Check sheet for the drawn part. Datum: minimum x, y, z corner. Units: mm. Coordinates: 2 decimals unless noted, no trailing zeros. Loops run counter-clockwise (first coordinate to the right, second up) from the corner with the lowest first, then second, coordinate; pieces in that order, holes last.
Q1. Sectioned sample at C-C (y = 7.5). Count the separate pieces of the cut face and the enclosed holes in it, then the cut area to 3 significant figures.
Q2. Material ranges on probe 1 along Z at (x, y) = (135, 7) (1 decimal); probe 2 along X at (y, z) = (9.5, 160) (1 decimal); probe 3 along Z at (x, y) = (17.5, 6.5), recorded low to high.
Q3. Sectioned sample at B-B (z = 25). Enter the section's corners in (x, y) (1 decimal), then the cut area to 3 significant figures.
Q4. Sectioned sample at D-D (x = 217). Enter the section's corners in (y, z), then the cut area to 3 significant figures.
Q5. Sectioned sample at A-A (x = 135). Enter the section's corners in (y, z) (1 decimal), then the cut area to 3 significant figures.
Q6. Go/stop test with flat-tipped pins: P1, Ø6, axis at x = 189, y = 5.5, coming from the +Z side; P2, Ø1.5, axis at y = 2, z = 192.5, coming from the -X side; P3, Ø3, axis at x = 69, y = 5.5, coming from the +Z side. Record where each tip stops, or that it passes through.
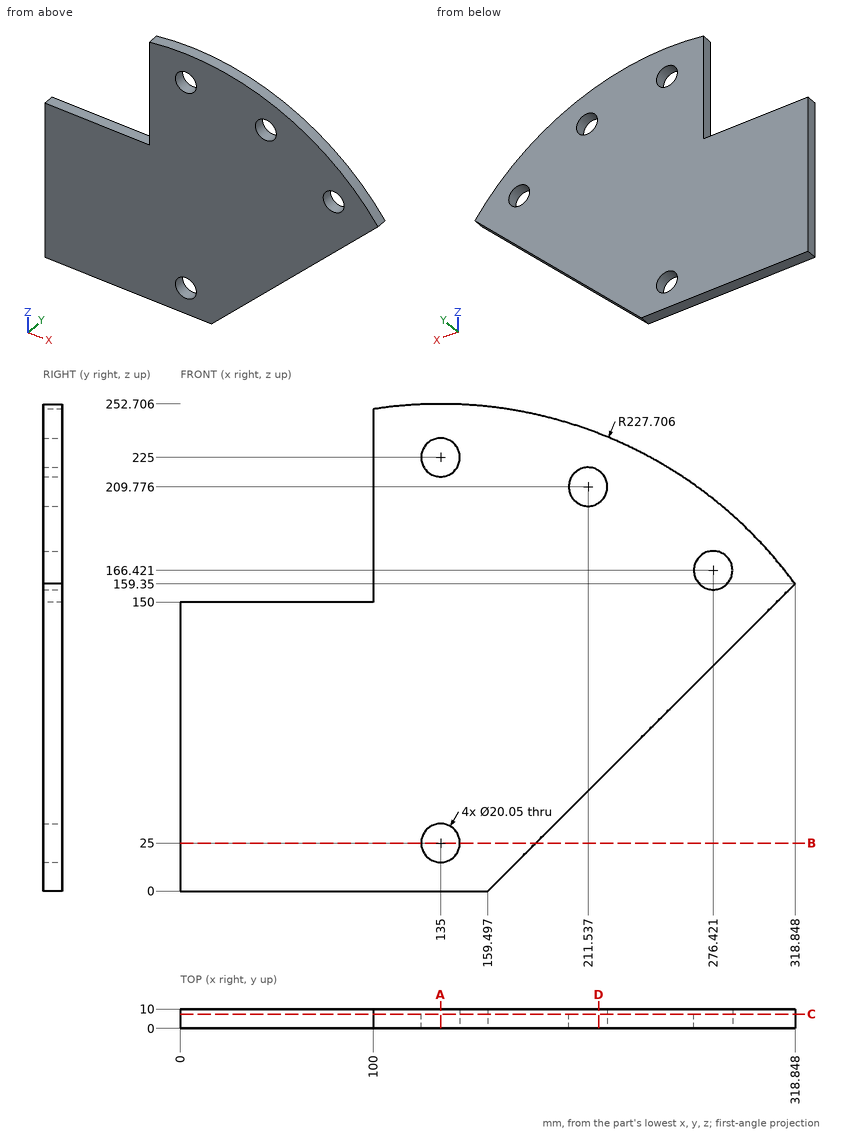
Geometry check:
1. separate pieces: 1
1. enclosed holes: 4
1. area: 51,200 mm2
2. probe 1: z = 0 to 15, 35 to 215, 235 to 252.7
2. probe 2: x = 100 to 268.7, 284.1 to 318.4
2. probe 3: z = 0 to 150
3. outline: (0, 0) - (125, 0) - (125, 10) - (0, 10) - close; (145, 0) - (184.5, 0) - (184.5, 10) - (145, 10) - close
3. area: 1,640 mm2
4. outline: (0, 57.5) - (10, 57.5) - (10, 201.37) - (0, 201.37) - close; (0, 218.18) - (10, 218.18) - (10, 237.43) - (0, 237.43) - close
4. area: 1,630 mm2
5. outline: (0, 0) - (10, 0) - (10, 15) - (0, 15) - close; (0, 35) - (10, 35) - (10, 215) - (0, 215) - close; (0, 235) - (10, 235) - (10, 252.7) - (0, 252.7) - close
5. area: 2,130 mm2
6. P1: stops at z = 246.92
6. P2: stops at x = 100
6. P3: stops at z = 150
